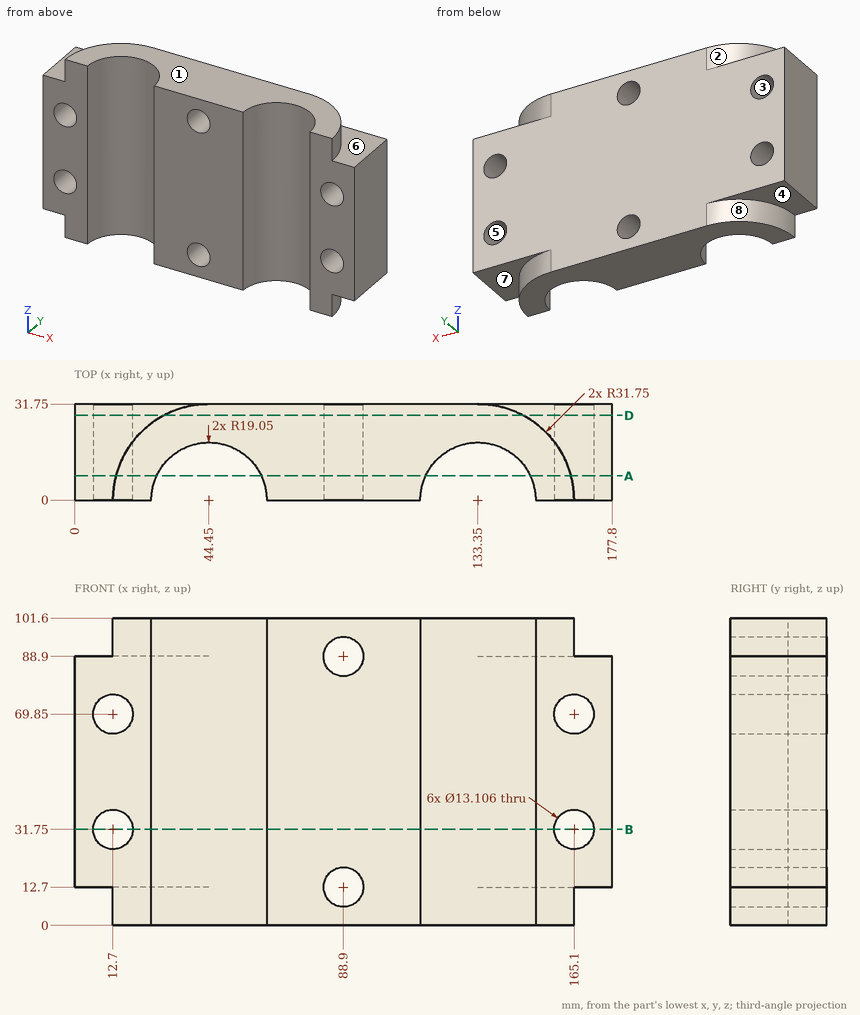
Answer from the drawing. Dimensions are ordinates in mm from the lowest x, y and z of the part. A direction names the side the tool comes from. Coordinates: 2 decimals unless noted, no trailing zeros. Order: outer loops, then holes, each group sorted by start corner. A loop starts at its lowest first (then second) coordinate and runs counter-clockwise, first axis right, second up. Notation, with made-up numbers: (63.5, -25) - (74.5, -25) arc R19 cw to (74.5, 9) - close; hole circle Ø9 at (71.25, 40.5). An arc over 180 degrees is marked (long way). Use one line per item in the form item = value.
(1) Section B-B, the plane z = 31.75 is taken. Give the vertices of the cut face in (x, y).
Computed values:
outline = (0, 0) - (6.15, 0) - (6.15, 31.75) - (0, 31.75) - close; (19.25, 0) - (25.4, 0) arc R19.05 cw to (63.5, 0) - (114.3, 0) arc R19.05 cw to (152.4, 0) - (158.55, 0) - (158.55, 31.75) - (19.25, 31.75) - close; (171.65, 0) - (177.8, 0) - (177.8, 31.75) - (171.65, 31.75) - close
(2) Section A-A, the plane y = 8 is taken. Give the number of separate pieces and of enclosed holes in the cut face, then the cut area to 3 significant figures.
Computed values:
separate_pieces = 3
enclosed_holes = 6
area = 9,530 mm²
(3) Given pin 1 Ø10.5 at (x, z) = (88.9, 88.9) entering from +Y, flat-ended and moving along its own axis, determine where the tip first touches the part or whether it passes through.
Computed values:
pin_1 = through
(4) Which of the six approach directions +Z, -Z, +X, -X, +Y, -Y give full straight-line access (tool end or side, diameter ignored) to the marked faces 5, 6, 7 and 8?
Computed values:
face_5 = +Y, -Y
face_6 = +Z, +X, +Y
face_7 = -Z, +X, +Y
face_8 = -Z, -X, +Y
(5) Straight lines are drawn through the part: L1, parallel to Z at x = 165.1, y = 12.5; L2, parallel to X at y = 4, z = 88 (1 decimal); L3, parallel to X at y = 28.5, z = 33.5 (1 decimal). For each, find the intervals that lie inside material, in ascending order.
Computed values:
L1 = 12.7 to 25.2, 38.3 to 63.3, 76.4 to 88.9
L2 = 0 to 25.8, 63.1 to 82.4, 95.4 to 114.7, 152 to 177.8
L3 = 0 to 6.4, 19 to 158.8, 171.4 to 177.8
(6) For a pull along Z with two mould halves and no side action, classify the marked faces 1, 2, 3 and 4 as pulls with the +Z half, pulls with the -Z half, needs draft (parallel to the pull), parting line crosses it, or undercut.
Computed values:
face_1 = pulls with the +Z half
face_2 = needs draft
face_3 = undercut
face_4 = pulls with the -Z half
(7) Section D-D, the plane y = 28 is taken. Give the vertices of the cut face in (x, z), then the cut area to 3 significant figures.
Computed values:
outline = (0, 12.7) - (29.48, 12.7) - (29.48, 0) - (148.32, 0) - (148.32, 12.7) - (177.8, 12.7) - (177.8, 88.9) - (148.32, 88.9) - (148.32, 101.6) - (29.48, 101.6) - (29.48, 88.9) - (0, 88.9) - close; hole circle Ø13.11 at (12.7, 31.75); hole circle Ø13.11 at (12.7, 69.85); hole circle Ø13.11 at (88.9, 12.7); hole circle Ø13.11 at (88.9, 88.9); hole circle Ø13.11 at (165.1, 31.75); hole circle Ø13.11 at (165.1, 69.85)
area = 15,800 mm²
